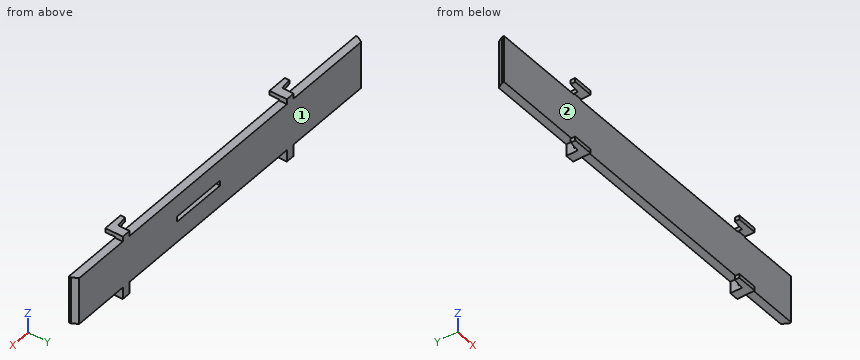
from build123d import *
from OCP.BRepFilletAPI import BRepFilletAPI_MakeChamfer

# Parameters (mm, degrees)
THICKNESS_EXTRUDE_DEPTH     = 3.5
HOOK_1_EXTRUDE_DEPTH        = 0.9
HOOK_START                  = -26.75
HOOK_2_EXTRUDE_DEPTH        = 0.9
HOOK_PATTERN_COUNT          = 2
HOOK_PATTERN_PITCH          = 96
HANDLE_SKETCH_W             = 25.4
HANDLE_SKETCH_H             = 2.35
HANDLE_SLOT_CUT_DEPTH       = 3
HANDLE_SLOT_CHAMFER_1_SIZE  = 1.175
HANDLE_SLOT_CHAMFER_1_SIZE2 = 2.836700936
END_CHAMFERS_SIZE           = 2.6
END_CHAMFERS_SIZE2          = 1.5011107


with BuildPart() as part:
    # Top Sketch → Thickness Extrude (new body)
    with BuildSketch(Plane(origin=(0, 0, 0), x_dir=(1, 0, 0), z_dir=(0, 1, 0))):
        Polygon((-27, -11), (-27, -12.375), (-31, -12.375), (-31, -11), (-123, -11), (-123, -12.375), (-127, -12.375), (-127, -11), (-168, -11), (-168, 10), (-127, 10), (-127, 14.375), (-123, 14.375), (-123, 10), (-31, 10), (-31, 14.375), (-27, 14.375), (-27, 10), (0, 10), (0, -11), align=None)
    extrude(amount=THICKNESS_EXTRUDE_DEPTH)


with BuildPart() as body_2:
    # Hook Sketch → Hook 1 Extrude (new, symmetric)
    with BuildSketch(Plane.XY.offset(12.375)):
        Polygon((-31, 3.5), (-27, 3.5), (-27, -4.258262488), (-36, -4.258262488), (-36, -2.258262488), (-31, -1.6), align=None)
    hook_1_extrude = extrude(amount=HOOK_1_EXTRUDE_DEPTH, both=True)


with BuildPart() as body_3:
    # Hook Sketch<2> → Hook 2 Extrude (new, symmetric)
    with BuildSketch(Plane.XY.offset(12.375).offset(HOOK_START)):
        Polygon((-31, 3.5), (-27, 3.5), (-27, -4.258262488), (-36, -4.258262488), (-36, -2.258262488), (-31, -1.6), align=None)
    hook_2_extrude = extrude(amount=HOOK_2_EXTRUDE_DEPTH, both=True)


with BuildPart() as hook_pattern_1:
    # Hook Pattern: pattern copy
    add(hook_1_extrude.moved(Location(Vector(-1, 0, 0) * (1 * HOOK_PATTERN_PITCH))))


with BuildPart() as hook_pattern_2:
    # Hook Pattern: pattern copy
    add(hook_2_extrude.moved(Location(Vector(-1, 0, 0) * (1 * HOOK_PATTERN_PITCH))))


with BuildPart() as part_1:
    add(part.part)

    # Combine Bodies: union body 2, body 3, Hook Pattern_1, Hook Pattern_2
    add(body_2.part)
    add(body_3.part)
    add(hook_pattern_1.part)
    add(hook_pattern_2.part)

    # Handle Sketch → Handle Slot Cut (cut)
    with BuildSketch(Plane(origin=(0, 3.5, 0), x_dir=(1, 0, 0), z_dir=(0, 1, 0))):
        with Locations((-71.3, -0.5)):
            Rectangle(HANDLE_SKETCH_W, HANDLE_SKETCH_H)
    extrude(amount=-HANDLE_SLOT_CUT_DEPTH, mode=Mode.SUBTRACT)

    # Handle Slot Chamfer 1
    handle_slot_chamfer_1_edges = [part_1.edges().sort_by_distance(p)[0] for p in [
        (-71.3, 0.5, 1.675),
    ]]
    handle_slot_chamfer_1_side = [part_1.faces().sort_by_distance(p)[0] for p in [
        (-71.3, 0.5, 0.5),
    ]]
    chamfer(handle_slot_chamfer_1_edges, length=HANDLE_SLOT_CHAMFER_1_SIZE, length2=HANDLE_SLOT_CHAMFER_1_SIZE2, reference=handle_slot_chamfer_1_side[0])

    # End Chamfers: one chamfer whose edges measure the first distance from different faces: ONE call of the kernel's chamfer builder (chamfer() names one face for all edges)
    end_chamfers_edges_1 = [part_1.edges().sort_by_distance(p)[0] for p in [
        (0, 3.5, 0.5),
    ]]
    end_chamfers_side_1 = [part_1.faces().sort_by_distance(p)[0] for p in [
        (0, 1.75, 0.5),
    ]]
    end_chamfers_edges_2 = [part_1.edges().sort_by_distance(p)[0] for p in [
        (-168, 3.5, 0.5),
    ]]
    end_chamfers_side_2 = [part_1.faces().sort_by_distance(p)[0] for p in [
        (-168, 1.75, 0.5),
    ]]
    end_chamfers = BRepFilletAPI_MakeChamfer(part_1.part.solid().wrapped)
    for e in end_chamfers_edges_1:
        end_chamfers.Add(END_CHAMFERS_SIZE, END_CHAMFERS_SIZE2, e.wrapped, end_chamfers_side_1[0].wrapped)  # the first distance lies on this face
    for e in end_chamfers_edges_2:
        end_chamfers.Add(END_CHAMFERS_SIZE, END_CHAMFERS_SIZE2, e.wrapped, end_chamfers_side_2[0].wrapped)  # the first distance lies on this face
    add(Compound.cast(end_chamfers.Shape()), mode=Mode.REPLACE)


solid = part_1.part
CAD build for the part. Positions are in the model's coordinates, mm. Face numbers are marked on the shaded views. Give positions to 0.01 mm unless a question says otherwise; leave off trailing zeros. Order: outer loops, then holes, each group sorted by start corner. A loop starts at its lowest first (then second) coordinate and runs counter-clockwise, first axis right, second up. Notation, with made-up numbers: (-4, 27) -> (53, 27) arc R19 cw to (53, 59) -> close; hole circle Ø10 at (-25.75, -16). An arc over 180 degrees is marked (long way). Return JSON: item names as keys, results as strings.
Q1. Saw through at B-B (x = -61). Write the cut outline in (y, z) (3 decimals).
Working result:
{"outline": "(0, -10) -> (3.5, -10) -> (3.5, -0.675) -> (0.5, -0.675) -> (0.5, 0.5) -> (3.337, 1.675) -> (3.5, 1.675) -> (3.5, 11) -> (0, 11) -> close"}
Q2. Saw through at C-C (x = -85.5). Write the cut outline in (y, z).
Working result:
{"outline": "(0, -10) -> (3.5, -10) -> (3.5, 11) -> (0, 11) -> close"}
Q3. Saw through at A-A (z = 9.5). Write the cut outline in (x, y), then the cut area to 3 significant figures.
Working result:
{"outline": "(-168, 0) -> (0, 0) -> (0, 0.9) -> (-1.5, 3.5) -> (-166.5, 3.5) -> (-168, 0.9) -> close", "area": "584 mm²"}
Q4. Flat gauge pins, fed straight in: pin 1 (0.7 mm diameter, centred on y = 0, z = 11.5, fed in from -X); pin 2 (0.9 mm diameter, centred on y = -3, z = 12, fed in from -X); pin 3 (0.7 mm diameter, centred on y = 2.5, z = 0.5, fed in from -X); pin 4 (3 mm diameter, centred on y = -2, z = -11.5, fed in from +X). Where does each tip first touch, or does it go through?
Working result:
{"pin 1": "x = -127", "pin 2": "x = -132", "pin 3": "x = -167.28", "pin 4": "through"}
Q5. Drill centre lines: line 1 (Y direction, x = -142, z = -5.25); line 2 (Z direction, x = -112.5, y = 1); line 3 (X direction, y = 2.25, z = 0). Where is each one in solid material? Low to high.
Working result:
{"line 1": "0 to 3.5", "line 2": "-10 to 11", "line 3": "-167.22 to -84, -58.6 to -0.78"}
Q6. Mould opens along Y. For the marked faces 1 and 2 say: pulls with the +Y half, pulls with the -Y half, needs draft (parallel to the pull), parting line crosses it, or undercut.
Working result:
{"face 1": "pulls with the +Y half", "face 2": "pulls with the -Y half"}
